from build123d import *

# Parameters (mm, degrees)
F0_W     = 40.1168912649
F0_H     = 26.2875333428
F1_DEPTH = 25.4
F2_SIZE  = 5.08
F3_R     = 10


with BuildPart() as f1:
    # F0 (on Front) → F1 (new body)
    with BuildSketch(Plane.XZ):
        with Locations((20.0584456325, 26.0967053473)):
            Rectangle(F0_W, F0_H)
    extrude(amount=F1_DEPTH)

    # F2
    f2_edges = [f1.edges().sort_by_distance(p)[0] for p in [
        (40.116891, 0, 26.096705),
        (20.058446, 0, 39.240472),
        (0, 0, 26.096705),
        (20.058446, 0, 12.952939),
    ]]
    chamfer(f2_edges, length=F2_SIZE)

    # F3
    f3_edges = [f1.edges().sort_by_distance(p)[0] for p in [
        (35.036891, 0, 26.096705),
        (20.058446, 0, 34.160472),
        (5.08, 0, 26.096705),
        (20.058446, 0, 18.032939),
    ]]
    fillet(f3_edges, radius=F3_R)


solid = f1.part
Source: CAD feature listing. Evaluate the final solid. Frame: model axes, mm. Coordinates: 2 decimals unless noted, no trailing zeros. Order: outer loops, then holes, each group sorted by start corner. A loop starts at its lowest first (then second) coordinate and runs counter-clockwise, first axis right, second up. Notation, with made-up numbers: M -27,-8.5 L 9,-8.5 A21 ccw 9,28.5 Z; hole C -20.75,64 d2. An arc over 180 degrees is marked long. Write each question's results on one line, items separated by ' | '. Start each with the question number.
Item 1: First-contact query: pin 1 Ø5 at (x, z) = (6.5, 29.5) entering from +Y. Flat tip, straight axial feed; report the tip coordinate or a pass-through.
Item 2: Cut plane B-B (z = 26.5). Return loops of the section in (x, y).
Item 3: Cut plane A-A (x = 27.5). Return loops of the section in (y, z).
Item 4: Line query: probe 1 along Z at (x, y) = (24, -4.25); probe 2 along Y at (x, z) = (31.5, 27.5); probe 3 along Y at (x, z) = (4, 33.25). Output: solid intervals per line, ascending.
Checked values:
1) pin 1: stops at y = 0
2) outline: M 0,-25.4 L 40.12,-25.4 L 40.12,-5.08 L 37.97,-2.93 A10 ccw 30.89,0 L 9.22,0 A10 ccw 2.15,-2.93 L 0,-5.08 Z
3) outline: M -25.4,12.95 L -5.08,12.95 L -2.93,15.1 A10 ccw 0,22.18 L 0,30.02 A10 ccw -2.93,37.09 L -5.08,39.24 L -25.4,39.24 Z
4) probe 1: z = 13.78 to 38.41 | probe 2: y = -25.4 to -0.02 | probe 3: y = -25.4 to -1.47
